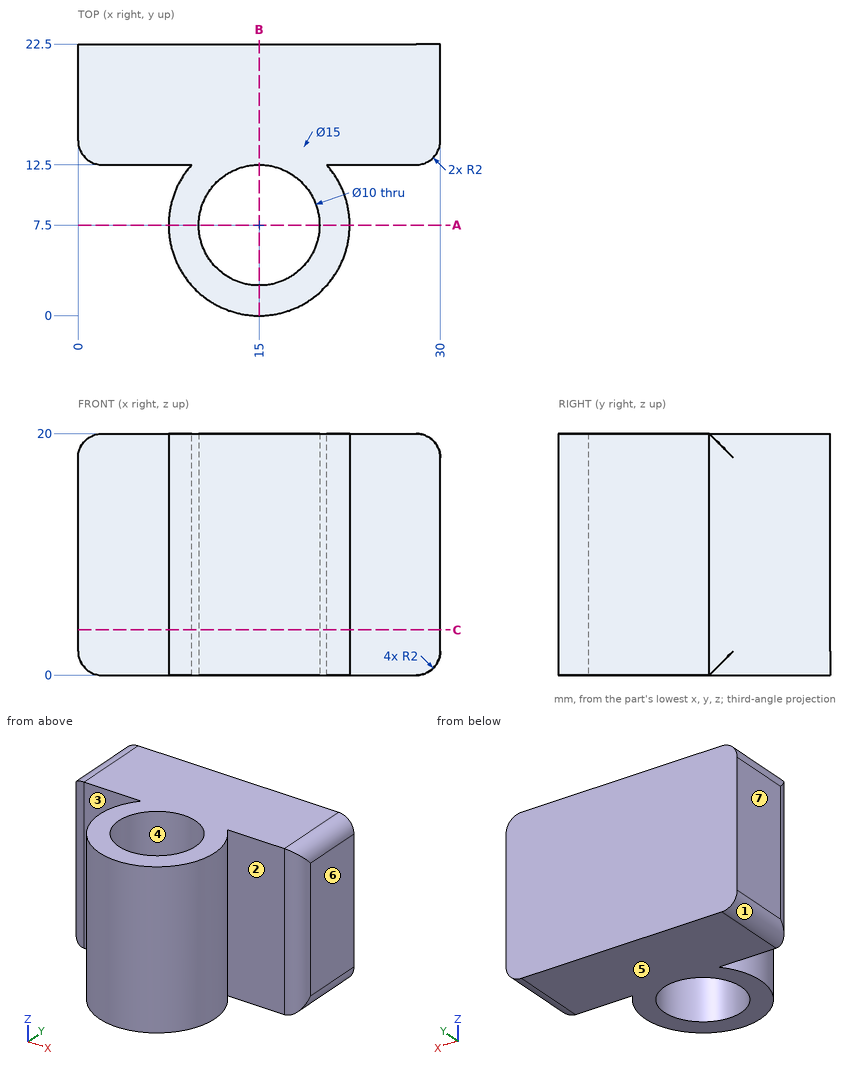
Geometry: see drawing. Coordinates: mm, zero at the bounding-box minimum. A direction names the side the tool comes from. Round coordinates to 2 decimals unless told otherwise and drop trailing zeros. Order: outer loops, then holes, each group sorted by start corner. A loop starts at its lowest first (then second) coordinate and runs counter-clockwise, first axis right, second up. Notation, with made-up numbers: (2.25, 59.5) -> (20.25, 59.5) arc R19 ccw to (20.25, 77.5) -> close; hole circle Ø11 at (12.25, 36). An arc over 180 degrees is marked (long way). Answer as CSV lines item,"result".
Item 1: Section A-A, the plane y = 7.5. Return loops of the section in (x, z), plus the area to 3 significant figures.
A:
outline,"(7.5, 0) -> (10, 0) -> (10, 20) -> (7.5, 20) -> close; (20, 0) -> (22.5, 0) -> (22.5, 20) -> (20, 20) -> close"
area,"100 mm²"
Item 2: Reachability of the marked faces 1, 2 and 3 from +Z, -Z, +X, -X, +Y, -Y: full face, straight path, thin tool, end or side. Return the list, or none.
A:
face 1,"-Z, -X, +Y, -Y"
face 2,"+Z, -Z, +X"
face 3,"+Z, -Z, -X"
Item 3: Pull-direction query (X, two-part tool) for the marked faces 4, 5, 6 and 7; classes: pulls with the +X half, pulls with the -X half, needs draft (parallel to the pull), parting line crosses it, or undercut.
A:
face 4,"undercut"
face 5,"needs draft"
face 6,"pulls with the +X half"
face 7,"pulls with the -X half"
Item 4: Pin query (flat end, axial travel): pin 1 Ø1.5 at (y, z) = (3.5, 16) entering from +X; pin 2 Ø8 at (y, z) = (12.5, 14) entering from -X; pin 3 Ø5 at (x, y) = (25.5, 9.5) entering from +Z; pin 4 Ø6 at (x, z) = (24.5, 11) entering from -Y. Return the tip coordinate at first contact, or that it passes through.
A:
pin 1,"x = 21.76"
pin 2,"x = 0"
pin 3,"through"
pin 4,"y = 3.76"
Item 5: Section C-C, the plane z = 3.75. Return loops of the section in (x, y), plus the area to 3 significant figures.
A:
outline,"(0, 14.5) arc R2 ccw to (2, 12.5) -> (9.41, 12.5) arc R7.5 ccw (long way) to (20.59, 12.5) -> (28, 12.5) arc R2 ccw to (30, 14.5) -> (30, 22.5) -> (0, 22.5) -> close; hole circle Ø10 at (15, 7.5)"
area,"377 mm²"
Item 6: Section B-B, the plane x = 15. Return loops of the section in (y, z), plus the area to 3 significant figures.
A:
outline,"(0, 0) -> (2.5, 0) -> (2.5, 20) -> (0, 20) -> close; (12.5, 0) -> (22.5, 0) -> (22.5, 20) -> (12.5, 20) -> close"
area,"250 mm²"
Item 7: Line query: L1, parallel to X at y = 7.5, z = 6.75; L2, parallel to Y at x = 27.75, z = 15; L3, parallel to Y at x = 16.25, z = 10. Output: solid intervals per line, ascending.
A:
L1,"7.5 to 10, 20 to 22.5"
L2,"12.5 to 22.5"
L3,"0.1 to 2.66, 12.34 to 22.5"
